Read the model definition and answer for the solid it produces. Units are mm, in the model's axes. A direction names the side the tool comes from. Round coordinates to 2 decimals unless told otherwise and drop trailing zeros. Loops run counter-clockwise (first coordinate to the right, second up) from the corner with the lowest first, then second, coordinate; pieces in that order, holes last. Notation, with made-up numbers: (-33, 57.5) - (-1, 57.5) arc R15 ccw to (-1, 82.5) - close; hole circle Ø11 at (32, 73.25). An arc over 180 degrees is marked (long way). Answer as CSV lines item,"result".
```python
from build123d import *

# Parameters (mm, degrees)
F0_W     = 5.5
F0_H     = 8
F0_W_2   = 3.3
F0_H_2   = 5
F1_DEPTH = 4
F2_R     = 1
F3_R     = 1
F4_R     = 0.5
F5_SIZE  = 0.5


with BuildPart() as f1:
    # F0 (on Top) → F1 (new body)
    with BuildSketch(Plane.XY):
        Rectangle(F0_W, F0_H)
        Rectangle(F0_W_2, F0_H_2, mode=Mode.SUBTRACT)
    extrude(amount=F1_DEPTH)

    # F2
    f2_edges = [f1.edges().sort_by_distance(p)[0] for p in [
        (-2.75, -4, 2),
        (2.75, -4, 2),
        (-2.75, 4, 2),
        (2.75, 4, 2),
    ]]
    fillet(f2_edges, radius=F2_R)

    # F3
    f3_edges = [f1.edges().sort_by_distance(p)[0] for p in [
        (1.65, 2.5, 2),
        (1.65, -2.5, 2),
        (-1.65, -2.5, 2),
        (-1.65, 2.5, 2),
    ]]
    fillet(f3_edges, radius=F3_R)

    # F4
    f4_edges = [f1.edges().sort_by_distance(p)[0] for p in [
        (1.65, 0, 4),
        (1.357107, 2.207107, 4),
        (1.357107, -2.207107, 4),
        (0, 2.5, 4),
        (0, -2.5, 4),
        (-1.357107, 2.207107, 4),
        (-1.357107, -2.207107, 4),
        (-1.65, 0, 4),
        (0, -4, 4),
        (-2.457107, -3.707107, 4),
        (2.457107, -3.707107, 4),
        (-2.75, 0, 4),
        (2.75, 0, 4),
        (-2.457107, 3.707107, 4),
        (2.457107, 3.707107, 4),
        (0, 4, 4),
    ]]
    fillet(f4_edges, radius=F4_R)

    # F5
    f5_edges = [f1.edges().sort_by_distance(p)[0] for p in [
        (1.65, 0, 0),
        (1.357107, 2.207107, 0),
        (1.357107, -2.207107, 0),
        (0, 2.5, 0),
        (0, -2.5, 0),
        (-1.357107, 2.207107, 0),
        (-1.357107, -2.207107, 0),
        (-1.65, 0, 0),
        (0, -4, 0),
        (-2.457107, -3.707107, 0),
        (2.457107, -3.707107, 0),
        (-2.75, 0, 0),
        (2.75, 0, 0),
        (-2.457107, 3.707107, 0),
        (2.457107, 3.707107, 0),
        (0, 4, 0),
    ]]
    chamfer(f5_edges, length=F5_SIZE)


solid = f1.part
```
1) A cutting plane is placed at B-B, the plane x = -0.5. Determine the outline of the cut face in (y, z), plus the area to 3 significant figures.
Entries:
outline,"(-4, 0.5) - (-3.5, 0) - (-3, 0) - (-2.5, 0.5) - (-2.5, 3.5) arc R0.5 ccw to (-3, 4) - (-3.5, 4) arc R0.5 ccw to (-4, 3.5) - close; (2.5, 0.5) - (3, 0) - (3.5, 0) - (4, 0.5) - (4, 3.5) arc R0.5 ccw to (3.5, 4) - (3, 4) arc R0.5 ccw to (2.5, 3.5) - close"
area,"11.3 mm^2"
2) A cutting plane is placed at C-C, the plane z = 2.9. Determine the outline of the cut face in (x, y).
Entries:
outline,"(-2.75, -3) arc R1 ccw to (-1.75, -4) - (1.75, -4) arc R1 ccw to (2.75, -3) - (2.75, 3) arc R1 ccw to (1.75, 4) - (-1.75, 4) arc R1 ccw to (-2.75, 3) - close; hole (-1.65, -1.5) arc R1 ccw to (-0.65, -2.5) - (0.65, -2.5) arc R1 ccw to (1.65, -1.5) - (1.65, 1.5) arc R1 ccw to (0.65, 2.5) - (-0.65, 2.5) arc R1 ccw to (-1.65, 1.5) - close"
3) The mould has two halves that part along X. Classify faces 4 (the face through (-1.48, 2.35, 0.31)), 5 (the face through (0, -4, 2)), 6 (the face through (-2.465, -3.699, 2.021)): pulls with the +X half, pulls with the -X half, needs draft (parallel to the pull), parting line crosses it, or undercut.
Entries:
face 4,"undercut"
face 5,"needs draft"
face 6,"pulls with the -X half"
4) This flat-tipped pin is pushed along its axis until it touches: P1, Ø2, axis at x = 1, y = -0.5, coming from the -Z side. Where does it stop, or does it pass through?
Entries:
P1,"stops at z = 0.15"
5) A cutting plane is placed at A-A, the plane y = 0.5. Determine the outline of the cut face in (x, z).
Entries:
outline,"(-2.75, 0.5) - (-2.25, 0) - (-2.15, 0) - (-1.65, 0.5) - (-1.65, 3.5) arc R0.5 ccw to (-2.15, 4) - (-2.25, 4) arc R0.5 ccw to (-2.75, 3.5) - close; (1.65, 0.5) - (2.15, 0) - (2.25, 0) - (2.75, 0.5) - (2.75, 3.5) arc R0.5 ccw to (2.25, 4) - (2.15, 4) arc R0.5 ccw to (1.65, 3.5) - close"
6) Find the intervals of material crossed by line 1 (X direction, y = -1, z = 1.15); line 2 (Y direction, x = 0.1, z = 1.95); line 3 (Y direction, x = -1.2, z = 2.05), in increasing order.
Entries:
line 1,"x = -2.75 to -1.65, 1.65 to 2.75"
line 2,"y = -4 to -2.5, 2.5 to 4"
line 3,"y = -4 to -2.34, 2.34 to 4"
7) A tool of negligible diameter and unlimited length cuts with its end or side. For faces 1 (the face through (-1.349, 2.215, 2.021)), 2 (the face through (2.24, -3.5, 0.2)), 3 (the face through (1.5, 2.33, 0.31)), from which of +Z, -Z, +X, -X, +Y, -Y can it reach the whole face along a straight path? Write none if from no direction.
Entries:
face 1,"+Z, -Z"
face 2,"-Z, +X, -Y"
face 3,"-Z"
